Verification items for the finished model (mm, model axes). Face numbers are marked on the shaded views. A direction names the side the tool comes from. Coordinates: 2 decimals unless noted, no trailing zeros. Loops run counter-clockwise (first coordinate to the right, second up) from the corner with the lowest first, then second, coordinate; pieces in that order, holes last. Notation, with made-up numbers: (35, -35.5) - (49, -35.5) arc R12 ccw to (49, -31.5) - close; hole circle Ø11 at (24, -17.5). An arc over 180 degrees is marked (long way). Answer as CSV lines item,"result". Start each with the question number.
1. Cross-section at C-C (x = -32). Enter the section's corners in (y, z), plus the area to 3 significant figures.
2. Cross-section at B-B (y = -29). Enter the section's corners in (x, z).
3. Gauge pin test, flat ends, axial feed: P1, Ø1.5, axis at x = 14.5, z = 5, coming from the -Y side; P2, Ø12, axis at x = -7.5, y = 4.5, coming from the -Z side; P3, Ø8, axis at x = -10, z = 18.5, coming from the +Y side. Record the tip position at first contact, or that the pin passes through.
4. Cross-section at D-D (y = 4). Enter the section's corners in (x, z), plus the area to 4 significant figures.
5. Set-up check for the marked faces 4, 5 and 6: record each of +Z, -Z, +X, -X, +Y, -Y from which the full face is reachable in a straight line by a thin tool's end or side.
6. Material ranges on line 1 (Y direction, x = -36.5, z = 7.75); line 2 (X direction, y = 31, z = 17); line 3 (Y direction, x = -29.5, z = 15.5), recorded low to high. Write a range as [from, to].
7. Release check for a two-part mould opening along X. For the marked faces 1, 2 and 3 record: pulls with the +X half, pulls with the -X half, needs draft (parallel to the pull), parting line crosses it, or undercut.
8. Cross-section at A-A (x = 36). Enter the section's corners in (y, z).
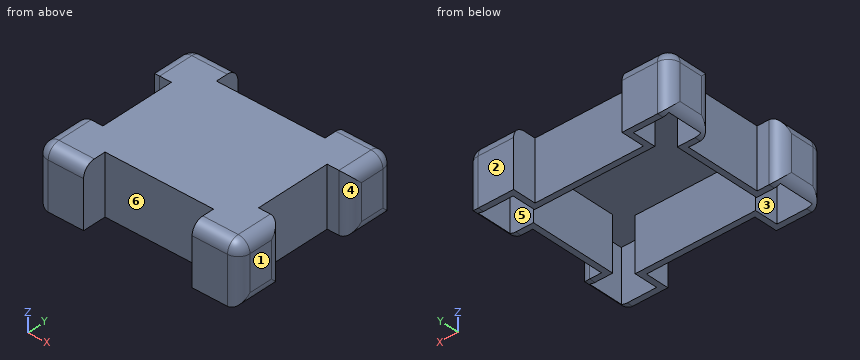
```python
from build123d import *

# Parameters (mm, degrees)
F0_W         = 10
F0_H         = 10
F1_DEPTH     = 25
F2_T         = -2.5
F3_T1_DEPTH  = 27.5
F3_T3_DEPTH  = 27.5
F3_T5_DEPTH  = 27.5
F3_T7_DEPTH  = 27.5
F3_T9_DEPTH  = 32.5
F3_T11_DEPTH = 50
F3_T13_DEPTH = 45
F3_T15_DEPTH = 45
F3_S19_W     = 5
F3_S19_H     = 5
F3_T20_DEPTH = 5
F3_S25_W     = 5
F3_S25_H     = 5
F3_T26_DEPTH = 5
F3_S31_W     = 5
F3_S31_H     = 5
F3_T32_DEPTH = 5
F3_S37_W     = 5
F3_S37_H     = 5
F3_T38_DEPTH = 5


# Not quite as in the source:
# - a fillet or chamfer that OpenCascade refuses, or shapes differently, is made with other operations: its cross-section is extruded or revolved along the edge and cut away or added


with BuildPart() as f1:
    # F0 (on Top) → F1 (new body)
    with BuildSketch(Plane.XY):
        Polygon((-33, 16), (-33, 26), (-23, 26), (-23, 36), (-43, 36), (-43, 16), align=None)
        with Locations((-28, 21)):
            Rectangle(F0_W, F0_H)
        Polygon((23, 26), (-23, 26), (-23, 16), (-33, 16), (-33, -16), (-23, -16), (-23, -26), (23, -26), (23, -16), (33, -16), (33, 16), (23, 16), align=None)
        Polygon((23, 36), (23, 26), (33, 26), (33, 16), (43, 16), (43, 36), align=None)
        with Locations((28, 21)):
            Rectangle(F0_W, F0_H)
        with Locations((-28, -21)):
            Rectangle(F0_W, F0_H)
        Polygon((-33, -26), (-33, -16), (-43, -16), (-43, -36), (-23, -36), (-23, -26), align=None)
        Polygon((43, -16), (33, -16), (33, -26), (23, -26), (23, -36), (43, -36), align=None)
        with Locations((28, -21)):
            Rectangle(F0_W, F0_H)
    extrude(amount=F1_DEPTH)

    # F2
    f2_openings = [f1.faces().sort_by_distance(p)[0] for p in [
        (0, 0, 0),
    ]]
    offset(amount=F2_T, openings=f2_openings, kind=Kind.INTERSECTION)

    # F3: fillet of radius 5 on 20 edges, made by hand

    # F3_s2 → F3_t1 (cut)
    with BuildSketch(Plane.YZ.offset(-38)):
        with BuildLine():
            ThreePointArc((36, 20), (34.5355339059, 23.5355339059), (31, 25))
            Line((31, 25), (36, 25))
            Line((36, 25), (36, 20))
        make_face()
        with BuildLine():
            ThreePointArc((-36, 20), (-34.5355339059, 23.5355339059), (-31, 25))
            Line((-31, 25), (-36, 25))
            Line((-36, 25), (-36, 20))
        make_face()
    extrude(amount=F3_T1_DEPTH, mode=Mode.SUBTRACT)

    # F3_s4 → F3_t3 (cut)
    with BuildSketch(Plane.YZ.offset(10.5)):
        with BuildLine():
            ThreePointArc((-36, 20), (-34.5355339059, 23.5355339059), (-31, 25))
            Line((-31, 25), (-36, 25))
            Line((-36, 25), (-36, 20))
        make_face()
        with BuildLine():
            ThreePointArc((36, 20), (34.5355339059, 23.5355339059), (31, 25))
            Line((31, 25), (36, 25))
            Line((36, 25), (36, 20))
        make_face()
    extrude(amount=F3_T3_DEPTH, mode=Mode.SUBTRACT)

    # F3_s6 → F3_t5 (cut)
    with BuildSketch(Plane.XZ.offset(-31)):
        with BuildLine():
            ThreePointArc((43, 20), (41.5355339059, 23.5355339059), (38, 25))
            Line((38, 25), (43, 25))
            Line((43, 25), (43, 20))
        make_face()
        with BuildLine():
            ThreePointArc((-43, 20), (-41.5355339059, 23.5355339059), (-38, 25))
            Line((-38, 25), (-43, 25))
            Line((-43, 25), (-43, 20))
        make_face()
    extrude(amount=F3_T5_DEPTH, mode=Mode.SUBTRACT)

    # F3_s8 → F3_t7 (cut)
    with BuildSketch(Plane.XZ.offset(3.5)):
        with BuildLine():
            ThreePointArc((43, 20), (41.5355339059, 23.5355339059), (38, 25))
            Line((38, 25), (43, 25))
            Line((43, 25), (43, 20))
        make_face()
        with BuildLine():
            ThreePointArc((-43, 20), (-41.5355339059, 23.5355339059), (-38, 25))
            Line((-38, 25), (-43, 25))
            Line((-43, 25), (-43, 20))
        make_face()
    extrude(amount=F3_T7_DEPTH, mode=Mode.SUBTRACT)

    # F3_s10 → F3_t9 (cut)
    with BuildSketch(Plane.XY.offset(-12.5)):
        with BuildLine():
            ThreePointArc((-38, 36), (-41.5355339059, 34.5355339059), (-43, 31))
            Line((-43, 31), (-43, 36))
            Line((-43, 36), (-38, 36))
        make_face()
        with BuildLine():
            ThreePointArc((43, 31), (41.5355339059, 34.5355339059), (38, 36))
            Line((38, 36), (43, 36))
            Line((43, 36), (43, 31))
        make_face()
        with BuildLine():
            ThreePointArc((38, -36), (41.5355339059, -34.5355339059), (43, -31))
            Line((43, -31), (43, -36))
            Line((43, -36), (38, -36))
        make_face()
        with BuildLine():
            ThreePointArc((-43, -31), (-41.5355339059, -34.5355339059), (-38, -36))
            Line((-38, -36), (-43, -36))
            Line((-43, -36), (-43, -31))
        make_face()
    extrude(amount=F3_T9_DEPTH, mode=Mode.SUBTRACT)

    # F3_s12 → F3_t11 (cut)
    with BuildSketch(Plane.XY.offset(-12.5)):
        with BuildLine():
            ThreePointArc((-43, 21), (-41.5355339059, 17.4644660941), (-38, 16))
            Line((-38, 16), (-43, 16))
            Line((-43, 16), (-43, 21))
        make_face()
        with BuildLine():
            ThreePointArc((38, 16), (41.5355339059, 17.4644660941), (43, 21))
            Line((43, 21), (43, 16))
            Line((43, 16), (38, 16))
        make_face()
        with BuildLine():
            ThreePointArc((43, -21), (41.5355339059, -17.4644660941), (38, -16))
            Line((38, -16), (43, -16))
            Line((43, -16), (43, -21))
        make_face()
        with BuildLine():
            ThreePointArc((-38, -16), (-41.5355339059, -17.4644660941), (-43, -21))
            Line((-43, -21), (-43, -16))
            Line((-43, -16), (-38, -16))
        make_face()
    extrude(amount=F3_T11_DEPTH, mode=Mode.SUBTRACT)

    # F3_s14 → F3_t13 (cut)
    with BuildSketch(Plane.XZ.offset(-48.5)):
        with BuildLine():
            ThreePointArc((-43, 5), (-41.5355339059, 1.4644660941), (-38, 0))
            Line((-38, 0), (-43, 0))
            Line((-43, 0), (-43, 5))
        make_face()
        with BuildLine():
            ThreePointArc((43, 5), (41.5355339059, 1.4644660941), (38, 0))
            Line((38, 0), (43, 0))
            Line((43, 0), (43, 5))
        make_face()
    extrude(amount=F3_T13_DEPTH, mode=Mode.SUBTRACT)

    # F3_s16 → F3_t15 (cut)
    with BuildSketch(Plane.XZ.offset(3.5)):
        with BuildLine():
            ThreePointArc((43, 5), (41.5355339059, 1.4644660941), (38, 0))
            Line((38, 0), (43, 0))
            Line((43, 0), (43, 5))
        make_face()
        with BuildLine():
            ThreePointArc((-43, 5), (-41.5355339059, 1.4644660941), (-38, 0))
            Line((-38, 0), (-43, 0))
            Line((-43, 0), (-43, 5))
        make_face()
    extrude(amount=F3_T15_DEPTH, mode=Mode.SUBTRACT)


with BuildPart() as f3_tool18:
    # F3_s19 → F3_t20 (new body)
    with BuildSketch(Plane.XZ.offset(-31)):
        with Locations((-40.5, 22.5)):
            Rectangle(F3_S19_W, F3_S19_H)
    extrude(amount=-F3_T20_DEPTH)

    # F3_s21 → F3_t22 (revolve, cut)
    with BuildSketch(Plane(origin=(-38, 31, 20), x_dir=(0.7071067812, 0, -0.7071067812), z_dir=(0.7071067812, 0, 0.7071067812))):
        with BuildLine():
            ThreePointArc((0, -5), (5, 0), (0, 5))
            Line((0, 5), (0, -5))
        make_face()
    revolve(axis=Axis((-38, 31, 20), (0, 1, 0)), mode=Mode.SUBTRACT)


with BuildPart() as f1_1:
    add(f1.part)

    # F3_t17: cut F3_tool18
    add(f3_tool18.part, mode=Mode.SUBTRACT)


with BuildPart() as f3_tool24:
    # F3_s25 → F3_t26 (new body)
    with BuildSketch(Plane.XY.offset(20)):
        with Locations((-40.5, -33.5)):
            Rectangle(F3_S25_W, F3_S25_H)
    extrude(amount=F3_T26_DEPTH)

    # F3_s27 → F3_t28 (revolve, cut)
    with BuildSketch(Plane(origin=(-38, -31, 20), x_dir=(0.7071067812, 0.7071067812, 0), z_dir=(0.7071067812, -0.7071067812, 0))):
        with BuildLine():
            ThreePointArc((0, -5), (5, 0), (0, 5))
            Line((0, 5), (0, -5))
        make_face()
    revolve(axis=Axis((-38, -31, 20), (0, 0, 1)), mode=Mode.SUBTRACT)


with BuildPart() as f1_2:
    add(f1_1.part)

    # F3_t23: cut F3_tool24
    add(f3_tool24.part, mode=Mode.SUBTRACT)


with BuildPart() as f3_tool30:
    # F3_s31 → F3_t32 (new body)
    with BuildSketch(Plane.XZ.offset(31)):
        with Locations((40.5, 22.5)):
            Rectangle(F3_S31_W, F3_S31_H)
    extrude(amount=F3_T32_DEPTH)

    # F3_s33 → F3_t34 (revolve, cut)
    with BuildSketch(Plane(origin=(38, -31, 20), x_dir=(-0.7071067812, 0, -0.7071067812), z_dir=(-0.7071067812, 0, 0.7071067812))):
        with BuildLine():
            ThreePointArc((0, -5), (5, 0), (0, 5))
            Line((0, 5), (0, -5))
        make_face()
    revolve(axis=Axis((38, -31, 20), (0, -1, 0)), mode=Mode.SUBTRACT)


with BuildPart() as f1_3:
    add(f1_2.part)

    # F3_t29: cut F3_tool30
    add(f3_tool30.part, mode=Mode.SUBTRACT)


with BuildPart() as f3_tool36:
    # F3_s37 → F3_t38 (new body)
    with BuildSketch(Plane.XZ.offset(-31)):
        with Locations((40.5, 22.5)):
            Rectangle(F3_S37_W, F3_S37_H)
    extrude(amount=-F3_T38_DEPTH)

    # F3_s39 → F3_t40 (revolve, cut)
    with BuildSketch(Plane(origin=(38, 31, 20), x_dir=(-0.7071067812, 0, -0.7071067812), z_dir=(0.7071067812, 0, -0.7071067812))):
        with BuildLine():
            ThreePointArc((0, -5), (5, 0), (0, 5))
            Line((0, 5), (0, -5))
        make_face()
    revolve(axis=Axis((38, 31, 20), (0, 1, 0)), mode=Mode.SUBTRACT)


with BuildPart() as f1_4:
    add(f1_3.part)

    # F3_t35: cut F3_tool36
    add(f3_tool36.part, mode=Mode.SUBTRACT)


solid = f1_4.part
```
Values follow:
1,outline,"(-36, 0) - (-33.5, 0) - (-33.5, 22.5) - (-18.5, 22.5) - (-18.5, 0) - (18.5, 0) - (18.5, 22.5) - (33.5, 22.5) - (33.5, 0) - (36, 0) - (36, 20) arc R5 ccw to (31, 25) - (-31, 25) arc R5 ccw to (-36, 20) - close"
1,area,"1,110 mm²"
2,outline,"(-43, 5) arc R5 ccw to (-40.5, 0.67) - (-40.5, 22.5) - (-25.5, 22.5) - (-25.5, 0) - (-23, 0) - (-23, 25) - (-38, 25) arc R5 ccw to (-43, 20) - close; (23, 0) - (25.5, 0) - (25.5, 22.5) - (40.5, 22.5) - (40.5, 0.67) arc R5 ccw to (43, 5) - (43, 20) arc R5 ccw to (38, 25) - (23, 25) - close"
3,P1,"stops at y = -26"
3,P2,"stops at z = 22.5"
3,P3,"stops at y = 26"
4,outline,"(-33, 0) - (-30.5, 0) - (-30.5, 22.5) - (30.5, 22.5) - (30.5, 0) - (33, 0) - (33, 25) - (-33, 25) - close"
4,area,"277.5 mm²"
5,face 4,"+Z, -Z, +X"
5,face 5,"-Z"
5,face 6,"+Z, -Z, -Y"
6,line 1,"y = [-36, -33.5], [-18.5, -16], [16, 18.5], [33.5, 36]"
6,line 2,"x = [-43, -40.5], [-25.5, -23], [23, 25.5], [40.5, 43]"
6,line 3,"y = [-36, -33.5], [33.5, 36]"
7,face 1,"pulls with the +X half"
7,face 2,"needs draft"
7,face 3,"undercut"
8,outline,"(-36, 0) - (-33.5, 0) - (-33.5, 22.5) - (-18.5, 22.5) - (-18.5, 0) - (-16, 0) - (-16, 25) - (-31, 25) arc R5 ccw to (-36, 20) - close; (16, 0) - (18.5, 0) - (18.5, 22.5) - (33.5, 22.5) - (33.5, 0) - (36, 0) - (36, 20) arc R5 ccw to (31, 25) - (16, 25) - close"
